Read the model definition and answer for the solid it produces. Units are mm, in the model's axes. Face numbers are marked on the shaded views. A direction names the side the tool comes from. Round coordinates to 2 decimals unless told otherwise and drop trailing zeros. Order: outer loops, then holes, each group sorted by start corner. A loop starts at its lowest first (then second) coordinate and runs counter-clockwise, first axis right, second up.
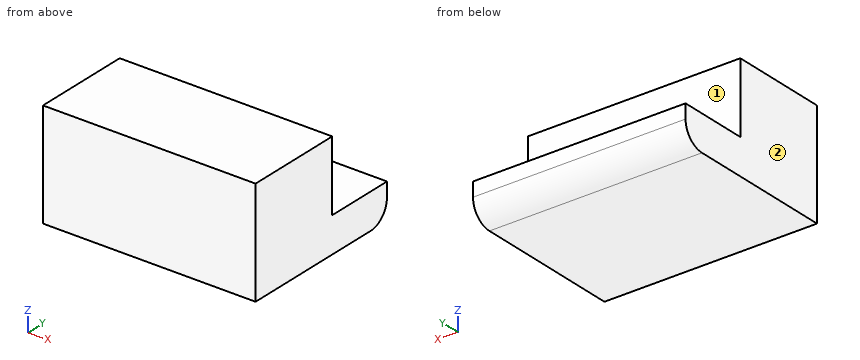
from build123d import *

# Parameters (mm, degrees)
SKETCH_1_W          = 30
SKETCH_1_H          = 24
EXTRUDE_1_DEPTH     = 15
SKETCH_2_W          = 30
SKETCH_2_H          = 10
CUT_EXTRUDE_1_DEPTH = 10
FILLET_1_R          = 3


with BuildPart() as part:
    # 草图1 → 凸台-拉伸1 (new body)
    with BuildSketch(Plane.XY):
        with Locations((-10.346525097, 8.485714286)):
            Rectangle(SKETCH_1_W, SKETCH_1_H)
    extrude(amount=EXTRUDE_1_DEPTH)

    # 草图2 → 切除-拉伸1 (cut)
    with BuildSketch(Plane.XY.offset(15)):
        with Locations((-10.346525097, 15.485714286)):
            Rectangle(SKETCH_2_W, SKETCH_2_H)
    extrude(amount=-CUT_EXTRUDE_1_DEPTH, mode=Mode.SUBTRACT)

    # 圆角1
    fillet_1_edges = [part.edges().sort_by_distance(p)[0] for p in [
        (-10.346525097, 20.485714286, 0),
    ]]
    fillet(fillet_1_edges, radius=FILLET_1_R)


solid = part.part
Q1. Flat-ended cylindrical pins translate along their axes: pin 1 (8 mm diameter, centred on x = -4, z = 13, fed in from +Y); pin 2 (5 mm diameter, centred on x = -17, y = 17.5, fed in from +Z). Find the tip coordinate at first contact, or state that the pin passes through.
Outcome:
pin 1: stops at y = 10.49
pin 2: stops at z = 5
Q2. For the marked faces 1 and 2, determine the directions among +Z, -Z, +X, -X, +Y, -Y from which every point of the face is accessible in a straight line to the end or side of a thin tool.
Outcome:
face 1: +Z, +X, -X, +Y
face 2: +Z, -Z, -X, +Y, -Y
Q3. A cutting plane is placed at A-A, the plane x = -22.75. Give the vertices of the cut face in (y, z), plus the area to 3 significant figures.
Outcome:
outline: (-3.51, 0) - (17.49, 0) arc R3 ccw to (20.49, 3) - (20.49, 5) - (10.49, 5) - (10.49, 15) - (-3.51, 15) - close
area: 258 mm2
Q4. A cutting plane is placed at B-B, the plane z = 10. Give the vertices of the cut face in (x, y).
Outcome:
outline: (-25.35, -3.51) - (4.65, -3.51) - (4.65, 10.49) - (-25.35, 10.49) - close
Q5. A cutting plane is placed at C-C, the plane y = 15.75. Give the vertices of the cut face in (x, z), plus the area to 3 significant figures.
Outcome:
outline: (-25.35, 0) - (4.65, 0) - (4.65, 5) - (-25.35, 5) - close
area: 150 mm2
Q6. Straight lines are drawn through the part: probe 1 along Y at (x, z) = (-3, 6.5); probe 2 along Z at (x, y) = (-23.75, 17.5); probe 3 along Y at (x, z) = (-4.25, 0.5). For each, find the intervals that lie inside material, in ascending order.
Outcome:
probe 1: y = -3.51 to 10.49
probe 2: z = 0 to 5
probe 3: y = -3.51 to 19.14
